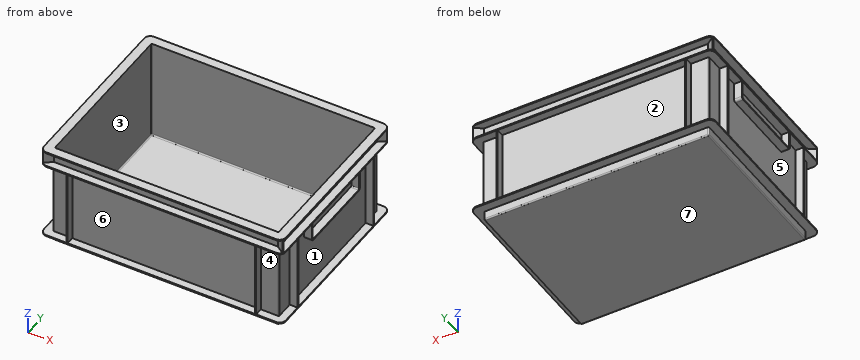
from build123d import *

# Parameters (mm, degrees)
F0_W      = 372
F0_H      = 272
F1_DEPTH  = 15
F2_W      = 372
F2_H      = 272
F3_DEPTH  = 2
F5_DEPTH  = 126
F7_DEPTH  = 2
F9_DEPTH  = 23
F11_DEPTH = 2
F12_W     = 370
F12_H     = 270
F13_DEPTH = 168
F15_DEPTH = 13
F17_DEPTH = 13
F18_R     = 2


with BuildPart() as f1:
    # F0 (on Top) → F1 (new body)
    with BuildSketch(Plane.XY):
        Rectangle(F0_W, F0_H)
    extrude(amount=F1_DEPTH)

    # F2 (on face) → F3 (join)
    with BuildSketch(Plane.XY.offset(15)):
        with BuildLine():
            Line((-190, -150), (190, -150))
            ThreePointArc((190, -150), (197.0710678119, -147.0710678119), (200, -140))
            Line((200, -140), (200, 140))
            ThreePointArc((200, 140), (197.0710678119, 147.0710678119), (190, 150))
            Line((190, 150), (-190, 150))
            ThreePointArc((-190, 150), (-197.0710678119, 147.0710678119), (-200, 140))
            Line((-200, 140), (-200, -140))
            ThreePointArc((-200, -140), (-197.0710678119, -147.0710678119), (-190, -150))
        make_face()
        Rectangle(F2_W, F2_H, mode=Mode.SUBTRACT)
        Rectangle(F2_W, F2_H)
    extrude(amount=F3_DEPTH)

    # F4 (on face) → F5 (join)
    with BuildSketch(Plane.XY.offset(17)):
        Polygon((157, -137), (187, -137), (187, -107), (200, -107), (200, -105), (187, -105), (187, 105), (200, 105), (200, 107), (187, 107), (187, 137), (157, 137), (157, 150), (155, 150), (155, 137), (-155, 137), (-155, 150), (-157, 150), (-157, 137), (-187, 137), (-187, 107), (-200, 107), (-200, 105), (-187, 105), (-187, -105), (-200, -105), (-200, -107), (-187, -107), (-187, -137), (-157, -137), (-157, -150), (-155, -150), (-155, -137), (155, -137), (155, -150), (157, -150), align=None)
    extrude(amount=F5_DEPTH)

    # F6 (on face) → F7 (join)
    with BuildSketch(Plane.XY.offset(143)):
        with BuildLine():
            Line((190, 150), (-190, 150))
            ThreePointArc((-190, 150), (-197.0710678119, 147.0710678119), (-200, 140))
            Line((-200, 140), (-200, -140))
            ThreePointArc((-200, -140), (-197.0710678119, -147.0710678119), (-190, -150))
            Line((-190, -150), (190, -150))
            ThreePointArc((190, -150), (197.0710678119, -147.0710678119), (200, -140))
            Line((200, -140), (200, 140))
            ThreePointArc((200, 140), (197.0710678119, 147.0710678119), (190, 150))
        make_face()
    extrude(amount=F7_DEPTH)

    # F8 (on face) → F9 (join)
    with BuildSketch(Plane.XY.offset(145)):
        with BuildLine():
            Line((-185.3079227659, -137), (185.3079227659, -137))
            Line((185.3079227659, -137), (197.8531877713, -146.1909160735))
            ThreePointArc((197.8531877713, -146.1909160735), (198.4340605379, -145.3727667773), (198.9300207482, -144.5005254622))
            Line((198.9300207482, -144.5005254622), (187, -135.7603498338))
            Line((187, -135.7603498338), (187, 135.7603498338))
            Line((187, 135.7603498338), (198.9300207482, 144.5005254622))
            ThreePointArc((198.9300207482, 144.5005254622), (198.4340605379, 145.3727667773), (197.8531877713, 146.1909160735))
            Line((197.8531877713, 146.1909160735), (185.3079227659, 137))
            Line((185.3079227659, 137), (-185.3079227659, 137))
            Line((-185.3079227659, 137), (-197.8531877713, 146.1909160735))
            ThreePointArc((-197.8531877713, 146.1909160735), (-198.4340605379, 145.3727667773), (-198.9300207482, 144.5005254622))
            Line((-198.9300207482, 144.5005254622), (-187, 135.7603498338))
            Line((-187, 135.7603498338), (-187, -135.7603498338))
            Line((-187, -135.7603498338), (-198.9300207482, -144.5005254622))
            ThreePointArc((-198.9300207482, -144.5005254622), (-198.4340605379, -145.3727667773), (-197.8531877713, -146.1909160735))
            Line((-197.8531877713, -146.1909160735), (-185.3079227659, -137))
        make_face()
    extrude(amount=F9_DEPTH)

    # F10 (on face) → F11 (join)
    with BuildSketch(Plane.XY.offset(168)):
        with BuildLine():
            Line((-190, -150), (190, -150))
            ThreePointArc((190, -150), (197.0710678119, -147.0710678119), (200, -140))
            Line((200, -140), (200, 140))
            ThreePointArc((200, 140), (197.0710678119, 147.0710678119), (190, 150))
            Line((190, 150), (-190, 150))
            ThreePointArc((-190, 150), (-197.0710678119, 147.0710678119), (-200, 140))
            Line((-200, 140), (-200, -140))
            ThreePointArc((-200, -140), (-197.0710678119, -147.0710678119), (-190, -150))
        make_face()
    extrude(amount=F11_DEPTH)

    # F12 (on face) → F13 (cut)
    with BuildSketch(Plane.XY.offset(170)):
        Rectangle(F12_W, F12_H)
    extrude(amount=-F13_DEPTH, mode=Mode.SUBTRACT)

    # F14 (on face) → F15 (join, through all)
    with BuildSketch(Plane(origin=(-187, 0, 0), x_dir=(0, -1, 0), z_dir=(-1, 0, 0))):
        with BuildLine():
            Line((-63, 111), (63, 111))
            ThreePointArc((63, 111), (65.8284271247, 112.1715728753), (67, 115))
            Line((67, 115), (67, 143))
            Line((67, 143), (65, 143))
            Line((65, 143), (65, 115))
            ThreePointArc((65, 115), (64.4142135624, 113.5857864376), (63, 113))
            Line((63, 113), (-63, 113))
            ThreePointArc((-63, 113), (-64.4142135624, 113.5857864376), (-65, 115))
            Line((-65, 115), (-65, 143))
            Line((-65, 143), (-67, 143))
            Line((-67, 143), (-67, 115))
            ThreePointArc((-67, 115), (-65.8284271247, 112.1715728753), (-63, 111))
        make_face()
    extrude(amount=F15_DEPTH)

    # F16 (on face) → F17 (join, through all)
    with BuildSketch(Plane.YZ.offset(187)):
        with BuildLine():
            ThreePointArc((63, 111), (65.8284271247, 112.1715728753), (67, 115))
            Line((67, 115), (67, 143))
            Line((67, 143), (65, 143))
            Line((65, 143), (65, 115))
            ThreePointArc((65, 115), (64.4142135624, 113.5857864376), (63, 113))
            Line((63, 113), (-63, 113))
            ThreePointArc((-63, 113), (-64.4142135624, 113.5857864376), (-65, 115))
            Line((-65, 115), (-65, 143))
            Line((-65, 143), (-67, 143))
            Line((-67, 143), (-67, 115))
            ThreePointArc((-67, 115), (-65.8284271247, 112.1715728753), (-63, 111))
            Line((-63, 111), (63, 111))
        make_face()
    extrude(amount=F17_DEPTH)

    # F18
    f18_edges = [f1.edges().sort_by_distance(p)[0] for p in [
        (-185, -135, 86),
        (185, -135, 86),
        (185, 135, 86),
        (0, 135, 2),
        (185, 0, 2),
        (0, -135, 2),
        (-185, 0, 2),
        (-185, 135, 86),
        (187, -137, 80),
        (187, 137, 80),
        (-187, 137, 80),
        (-187, -137, 80),
        (186, 0, 0),
        (0, 136, 0),
        (186, 136, 7.5),
        (0, -136, 0),
        (186, -136, 7.5),
        (-186, -136, 7.5),
        (-186, 0, 0),
        (-186, 136, 7.5),
    ]]
    fillet(f18_edges, radius=F18_R)


solid = f1.part
The model under review builds one solid part; all positions refer to its coordinate system, in mm. Face numbers are marked on the shaded views. A direction names the side the tool comes from. Coordinates: 2 decimals unless noted, no trailing zeros. Write each loop counter-clockwise with the first axis right and the second up, starting at its lowest first coordinate (ties: lowest second). Pieces come first, ordered by that corner, then holes. Notation, with made-up numbers: (33.5, 77.25) -> (45.5, 77.25) arc R23 cw to (45.5, 93.25) -> close; hole circle Ø3 at (27.5, -3). An arc over 180 degrees is marked (long way). Answer in a Markdown table with one row per item.
1. We need section A-A, the plane z = 156. State the section outline as (x, y) points, and give its area (3 significant figures).
Answers below:
| item | result |
|---|---|
| outline | (-198.93, -144.5) arc R10 ccw to (-197.85, -146.19) -> (-185.31, -137) -> (185.31, -137) -> (197.85, -146.19) arc R10 ccw to (198.93, -144.5) -> (187, -135.76) -> (187, 135.76) -> (198.93, 144.5) arc R10 ccw to (197.85, 146.19) -> (185.31, 137) -> (-185.31, 137) -> (-197.85, 146.19) arc R10 ccw to (-198.93, 144.5) -> (-187, 135.76) -> (-187, -135.76) -> close; hole (-185, -133) arc R2 ccw to (-183, -135) -> (183, -135) arc R2 ccw to (185, -133) -> (185, 133) arc R2 ccw to (183, 135) -> (-183, 135) arc R2 ccw to (-185, 133) -> close |
| area | 2,700 mm^2 |
2. For the marked faces 1, 2, 3 and 4, list the 3-axis set-ups (+Z, -Z, +X, -X, +Y, -Y) from which the entire face can be reached by the end or side of a thin tool; tool diameter is ignored.
Answers below:
| item | result |
|---|---|
| face 1 | +X |
| face 2 | +Y |
| face 3 | +Z |
| face 4 | +X, -Y |
3. Clearance check with flat-ended pins moving along their axes: pin 1 Ø14.5 at (x, z) = (-89.5, 6) entering from +Y; pin 2 Ø2 at (y, z) = (-39, 36.5) entering from +X; pin 3 Ø6.5 at (x, y) = (-190.5, -7) entering from -Z. State where each tip first meets the part, or that it passes through.
Answers below:
| item | result |
|---|---|
| pin 1 | stops at y = 136 |
| pin 2 | stops at x = 187 |
| pin 3 | stops at z = 15 |
4. Draft analysis for pull direction X (two halves, no side actions). For the marked faces 5, 6 and 7, state which applies: +X half, -X half, draft (parallel to the pull), parting line (faces both ways), or undercut.
Answers below:
| item | result |
|---|---|
| face 5 | -X half |
| face 6 | undercut |
| face 7 | draft |
5. Wall thickness on probe 1 along X at (y, z) = (-82, 35); probe 2 along Y at (x, z) = (42.5, 127); probe 3 along X at (y, z) = (28.5, 11.5): over which ranges is each line inside the solid? List them lowest first. Write a range as [from, to].
Answers below:
| item | result |
|---|---|
| probe 1 | x = [-187, -185], [185, 187] |
| probe 2 | y = [-137, -135], [135, 137] |
| probe 3 | x = [-186, -185], [185, 186] |
